Work out the finished part from the listing and answer in its coordinate system (mm). A direction names the side the tool comes from. Round coordinates to 2 decimals unless told otherwise and drop trailing zeros. Order: outer loops, then holes, each group sorted by start corner. A loop starts at its lowest first (then second) coordinate and runs counter-clockwise, first axis right, second up. Notation, with made-up numbers: (-9.5, 55.25) - (-1.5, 55.25) arc R19 ccw to (-1.5, 86.25) - close; hole circle Ø9 at (-3.75, 57.25). An arc over 180 degrees is marked (long way). Use one line per item in the form item = value. Start each with the question number.
Q1. For a pull along X with two mould halves and no side action, classify faces 5 (the flat face through (-0.1, -30, -0.4)), 6 (the cylindrical face through (0, -2, 15)), 7 (the flat face through (12, -2, 1)) as +X half, -X half, draft (parallel to the pull), parting line (faces both ways), or undercut.
Q2. The part is cut by section A-A on y = -46. Determine the outline of the cut face in (x, z).
Q3. The part is cut by section C-C on y = -26.25. Determine the outline of the cut face in (x, z).
Q4. Find the intervals of material crossed by line 1 (X direction, y = -4, z = -2); line 2 (Y direction, x = 2.75, z = -6); line 3 (Z direction, x = -0.25, y = -34.5), in increasing order. Write a range as [from, to].
Q5. Which of the six approach directions +Z, -Z, +X, -X, +Y, -Y give full straight-line access (tool end or side, diameter ignored) to faces 1 (the cylindrical face through (2.1, -27.75, -5.93)), 2 (the flat face through (0, -32, -6)), 3 (the cylindrical face through (-2.1, -25.25, -3.93)), 4 (the flat face through (0, -2, 2))?
Q6. The part is cut by section B-B on z = 5. Determine the outline of the cut face in (x, y), plus the area to 3 significant figures.
Q7. Given P1, Ø2.5, axis at x = 7, y = -1.5, coming from the -Z side; P2, Ø1.8, axis at y = -23.75, z = -4, coming from the -X side; P3, Ø4.5, axis at y = -18, z = -7.5, coming from the -X side, each flat-ended and moving along its own axis, determine where each tip first touches the part or whether it passes through.
from build123d import *

# Parameters (mm, degrees)
F1_DEPTH      = 5
F2_DEPTH      = 32
F3_R          = 1.5
F4_DEPTH      = 25
F5_DEPTH      = 25
F6_R          = 8
F7_DEPTH      = 25
F9_DEPTH      = 4.25
F9_DEPTH_BACK = 4.25
F10_R         = 1.5
F11_DEPTH     = 25


with BuildPart() as f1:
    # F0 (on Front) → F1 (new body)
    with BuildSketch(Plane.XZ):
        with BuildLine():
            Line((-8, 7), (-8, 2))
            Line((-8, 2), (-12, 2))
            Line((-12, 2), (-12, 0))
            Line((-12, 0), (-4.25, 0))
            Line((-4.25, 0), (0, 0))
            Line((0, 0), (4.25, 0))
            Line((4.25, 0), (12, 0))
            Line((12, 0), (12, 2))
            Line((12, 2), (8, 2))
            Line((8, 2), (8, 7))
            ThreePointArc((8, 7), (0, 15), (-8, 7))
        make_face()
        with BuildLine():
            ThreePointArc((3.316625, 12), (6, 7), (3.316625, 2))
            Line((3.316625, 2), (-3.316625, 2))
            ThreePointArc((-3.316625, 2), (-6, 7), (-3.316625, 12))
            Line((-3.316625, 12), (3.316625, 12))
        make_face(mode=Mode.SUBTRACT)
    extrude(amount=F1_DEPTH)

    # F0 (on Front) → F2 (join)
    with BuildSketch(Plane.XZ):
        Polygon((0, 0), (-4.25, 0), (-4.25, -8), (4.25, -8), (4.25, 0), align=None)
    extrude(amount=F2_DEPTH)

    # F3 (on Right) → F4 (cut)
    with BuildSketch(Plane.YZ):
        with Locations((-23.75, -4)):
            Circle(F3_R)
    extrude(amount=-F4_DEPTH, mode=Mode.SUBTRACT)

    # F3 (on Right) → F5 (cut)
    with BuildSketch(Plane.YZ):
        with Locations((-26.25, -6)):
            Circle(F3_R)
    extrude(amount=F5_DEPTH, mode=Mode.SUBTRACT)

    # F6 (on face) → F7 (cut)
    with BuildSketch(Plane.XZ.offset(5)):
        with Locations((0, 7)):
            Circle(F6_R)
    extrude(amount=F7_DEPTH, mode=Mode.SUBTRACT)

    # F8 (on Right) → F9 (join, two sides)
    with BuildSketch(Plane.YZ) as f9_sk:
        Polygon((-32, -8), (-32, -11.5), (-50, -11.5), (-50, -15.5), (-25, -15.5), (-17, -8), align=None)
    extrude(amount=F9_DEPTH)
    extrude(f9_sk.sketch, amount=-F9_DEPTH_BACK)

    # F10 (on face) → F11 (cut)
    with BuildSketch(Plane.XY.offset(-11.5)):
        with Locations((0, -46)):
            Circle(F10_R)
    extrude(amount=-F11_DEPTH, mode=Mode.SUBTRACT)


solid = f1.part
Found:
q1.face_5 = undercut
q1.face_6 = parting line
q1.face_7 = +X half
q2.outline = (-4.25, -15.5) - (-1.5, -15.5) - (-1.5, -11.5) - (-4.25, -11.5) - close; (1.5, -15.5) - (4.25, -15.5) - (4.25, -11.5) - (1.5, -11.5) - close
q3.outline = (-4.25, -15.5) - (4.25, -15.5) - (4.25, -7.5) - (0, -7.5) - (0, -4.5) - (4.25, -4.5) - (4.25, 0) - (3.87, 0) arc R8 cw to (-3.87, 0) - (-4.25, 0) - close
q4.line_1 = [-4.25, 4.25]
q4.line_2 = [-32, -27.75], [-24.75, 0]
q4.line_3 = [-15.5, -11.5]
q5.face_1 = +X
q5.face_2 = +Z, +X, -X, -Y
q5.face_3 = -X
q5.face_4 = +Y, -Y
q6.outline = (-8, -5) - (-5.66, -5) - (-5.66, 0) - (-8, 0) - close; (5.66, -5) - (8, -5) - (8, 0) - (5.66, 0) - close
q6.area = 23.4 mm²
q7.P1 = 0
q7.P2 = 0
q7.P3 = -4.25
